from build123d import *

# Parameters (mm, degrees)
F0_W      = 90
F0_H      = 32
F1_DEPTH  = 2
F2_W      = 4
F2_H      = 2
F3_DEPTH  = 6.5
F5_W      = 4
F5_H      = 2
F6_DEPTH  = 28
F4_W      = 4
F4_H      = 2
F7_DEPTH  = 28
F8_R      = 0.99999
F10_DEPTH = 15.25


# Not quite as in the source:
# - a fillet or chamfer is up to 0.001 mm smaller than in the source, because OpenCascade refuses the exact size


with BuildPart() as f1:
    # F0 (on Top) → F1 (new body)
    with BuildSketch(Plane.XY):
        with Locations((45, 16)):
            Rectangle(F0_W, F0_H)
    extrude(amount=F1_DEPTH)

    # F2 (on face) → F3 (join)
    with BuildSketch(Plane.XY.offset(2)):
        with Locations((2, 31)):
            Rectangle(F2_W, F2_H)
        with Locations((2, 1)):
            Rectangle(F2_W, F2_H)
        with Locations((88, 1)):
            Rectangle(F2_W, F2_H)
        with Locations((88, 31)):
            Rectangle(F2_W, F2_H)
    extrude(amount=F3_DEPTH)

    # F5 (on face) → F6 (join)
    with BuildSketch(Plane(origin=(0, 2, 0), x_dir=(-1, 0, 0), z_dir=(0, 1, 0))):
        with Locations((-2, 7.5)):
            Rectangle(F5_W, F5_H)
    extrude(amount=F6_DEPTH)

    # F4 (on face) → F7 (join)
    with BuildSketch(Plane(origin=(0, 2, 0), x_dir=(-1, 0, 0), z_dir=(0, 1, 0))):
        with Locations((-88, 7.5)):
            Rectangle(F4_W, F4_H)
    extrude(amount=F7_DEPTH)

    # F8 (radius 1 in the source; OpenCascade refuses exactly that, so slightly less here)
    f8_edges = [f1.edges().sort_by_distance(p)[0] for p in [
        (0, 16, 8.5),
        (4, 16, 8.5),
        (0, 32, 4.25),
        (0, 0, 4.25),
        (0, 16, 2),
        (2, 32, 8.5),
        (2, 0, 8.5),
        (0, 30, 4.25),
        (0, 2, 4.25),
        (4, 2, 4.25),
        (4, 30, 4.25),
        (4, 32, 5.25),
        (4, 0, 5.25),
        (86, 0, 5.25),
        (90, 0, 4.25),
        (86, 30, 4.25),
        (90, 30, 4.25),
        (86, 32, 5.25),
        (90, 32, 4.25),
        (90, 16, 8.5),
        (86, 16, 8.5),
        (88, 0, 8.5),
        (88, 32, 8.5),
        (90, 2, 4.25),
        (90, 16, 2),
    ]]
    fillet(f8_edges, radius=F8_R)

    # F9 (on face) → F10 (join)
    with BuildSketch(Plane(origin=(0, 0, 0), x_dir=(1, 0, 0), z_dir=(0, 0, -1))):
        Polygon((33.5, -30), (33.5, -25.5), (31.5, -25.5), (31.5, -32), (58.5, -32), (58.5, -25.5), (56.5, -25.5), (56.5, -30), align=None)
        Polygon((33.5, -21.5), (33.5, -17), (56.5, -17), (56.5, -21.5), (58.5, -21.5), (58.5, -15), (31.5, -15), (31.5, -21.5), align=None)
    extrude(amount=F10_DEPTH)


solid = f1.part
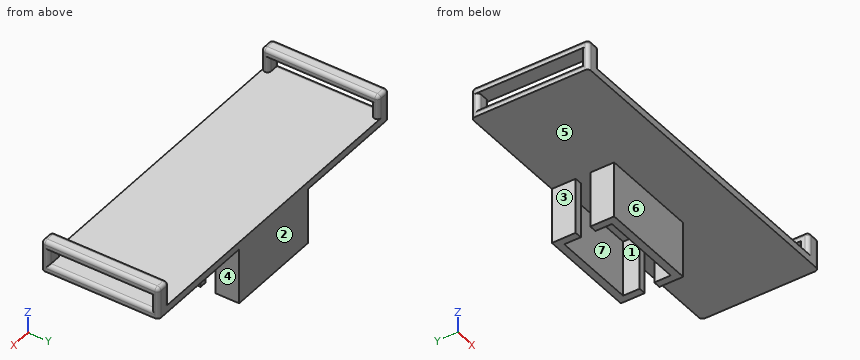
Read the model definition and answer for the solid it produces. Units are mm, in the model's axes. Face numbers are marked on the shaded views. A direction names the side the tool comes from. Coordinates: 2 decimals unless noted, no trailing zeros. Write each loop counter-clockwise with the first axis right and the second up, starting at its lowest first coordinate (ties: lowest second). Pieces come first, ordered by that corner, then holes. Notation, with made-up numbers: M 64,9 L 77,9 A37 cw 77,48 Z; hole C 78,51.5 d4. An arc over 180 degrees is marked long. Use a Markdown table: item, result.
Q1. The part is cut by section C-C, the plane z = 3.75. Give the number of separate pieces and of enclosed holes in the cut face, then the cut area to 3 significant figures.
Answer block:
| item | result |
|---|---|
| separate pieces | 4 |
| enclosed holes | 0 |
| area | 28.8 mm2 |
Q2. Straight lines are drawn through the part: L1, parallel to Y at x = 38.5, z = -8; L2, parallel to X at y = 21, z = -7.5; L3, parallel to X at y = 16, z = -12.75. For each, find the intervals that lie inside material, in ascending order. Write a range as [from, to].
Answer block:
| item | result |
|---|---|
| L1 | y = [15, 17], [30, 32] |
| L2 | x = [31.5, 33.5], [56.5, 58.5] |
| L3 | x = [31.5, 58.5] |
Q3. Each of these flat-tipped pins is pushed along its axis until it touches: pin 1 Ø2 at (y, z) = (28.5, -6) entering from -X; pin 2 Ø5 at (y, z) = (27.5, -4) entering from +X; pin 3 Ø12 at (x, y) = (41, 14.5) entering from +Z. Where does it stop, or does it pass through?
Answer block:
| item | result |
|---|---|
| pin 1 | stops at x = 31.5 |
| pin 2 | stops at x = 58.5 |
| pin 3 | stops at z = 2 |
Q4. Determine the mould class of the marked faces 4, 5, 6 and 7 for opening direction Y: released by +Y, released by -Y, zero draft, split by the parting line, or undercut.
Answer block:
| item | result |
|---|---|
| face 4 | zero draft |
| face 5 | undercut |
| face 6 | released by -Y |
| face 7 | undercut |
Q5. The part is cut by section B-B, the plane z = -11.75. Write down the section's boundary in (x, y), then the cut area to 3 significant figures.
Answer block:
| item | result |
|---|---|
| outline | M 31.5,15 L 58.5,15 L 58.5,21.5 L 56.5,21.5 L 56.5,17 L 33.5,17 L 33.5,21.5 L 31.5,21.5 Z; M 31.5,25.5 L 33.5,25.5 L 33.5,30 L 56.5,30 L 56.5,25.5 L 58.5,25.5 L 58.5,32 L 31.5,32 Z |
| area | 144 mm2 |
Q6. The part is cut by section A-A, the plane y = 20. Write down the section's boundary in (x, z), then the cut area to 3 significant figures.
Answer block:
| item | result |
|---|---|
| outline | M 0,0 L 31.5,0 L 31.5,-15.25 L 33.5,-15.25 L 33.5,0 L 56.5,0 L 56.5,-15.25 L 58.5,-15.25 L 58.5,0 L 90,0 L 90,1 A1 ccw 89,2 L 1,2 A1 ccw 0,1 Z; M 0,6.5 L 4,6.5 L 4,7.5 A1 ccw 3,8.5 L 1,8.5 A1 ccw 0,7.5 Z; M 86,6.5 L 90,6.5 L 90,7.5 A1 ccw 89,8.5 L 87,8.5 A1 ccw 86,7.5 Z |
| area | 256 mm2 |
Q7. The part is cut by section D-D, the plane x = 43. Write down the section's boundary in (y, z), then the cut area to 3 significant figures.
Answer block:
| item | result |
|---|---|
| outline | M 0,0 L 15,0 L 15,-15.25 L 17,-15.25 L 17,0 L 30,0 L 30,-15.25 L 32,-15.25 L 32,2 L 0,2 Z |
| area | 125 mm2 |
Q8. Which of the six approach directions +Z, -Z, +X, -X, +Y, -Y give full straight-line access (tool end or side, diameter ignored) to the marked faces 1, 2 and 3?
Answer block:
| item | result |
|---|---|
| face 1 | -Z |
| face 2 | +Z, -Z, +X, -X, +Y |
| face 3 | -Z, -X, +Y, -Y |
